Source: three-view drawing plus pictorial views. Frame: mm from the lowest corner of the part. A direction names the side the tool comes from. Give positions to 0.01 mm unless a question says otherwise; leave off trailing zeros. Loops run counter-clockwise (first coordinate to the right, second up) from the corner with the lowest first, then second, coordinate; pieces in that order, holes last. Notation, with made-up numbers: M 78.5,3.25 L 137.5,3.25 A18 cw 137.5,26.25 Z; hole C -30.75,10.5 d6. An arc over 180 degrees is marked long. One line per item, written item: value. Start each with the question number.
(1) Section D-D on z = 28.5. Output: boundary loops of the cut face in (x, y), plus the area to 3 significant figures.
(2) Section B-B on x = 18. Output: boundary loops of the cut face in (y, z).
(3) Section C-C on x = 25. Output: boundary loops of the cut face in (y, z), plus the area to 3 significant figures.
(4) Pin query (flat end, axial travel): P1, Ø6, axis at x = 15, z = 44, coming from the -Y side; P2, Ø1.5, axis at y = 25, z = 49, coming from the -X side; P3, Ø12, axis at y = 7, z = 25.5, coming from the +X side; P4, Ø4.5, axis at y = 5.5, z = 34, coming from the -X side. Return the tip coordinate at first contact, or that it passes through.
(5) Section A-A on z = 16. Output: boundary loops of the cut face in (x, y), plus the area to 3 significant figures.
(6) Ray query, line 1 along X through (y, z) = (42.7, 16); line 2 along Y through (x, z) = (4, 27); line 3 along Z through (x, y) = (18.5, 41.5). Return the intervals inside material, ascending. Write a range as from..to.
(7) Access query for the marked faces 5, 6, 7 and 8. Directions: +Z, -Z, +X, -X, +Y, -Y. A direction counts if a zero-diameter tool reaches every point of the face in a straight line with its end or side. Return the directions, or none.
(8) Pull-direction query (Y, two-part tool) for the marked faces 1, 2, 3 and 4; classes: released by +Y, released by -Y, zero draft, split by the parting line, or undercut.
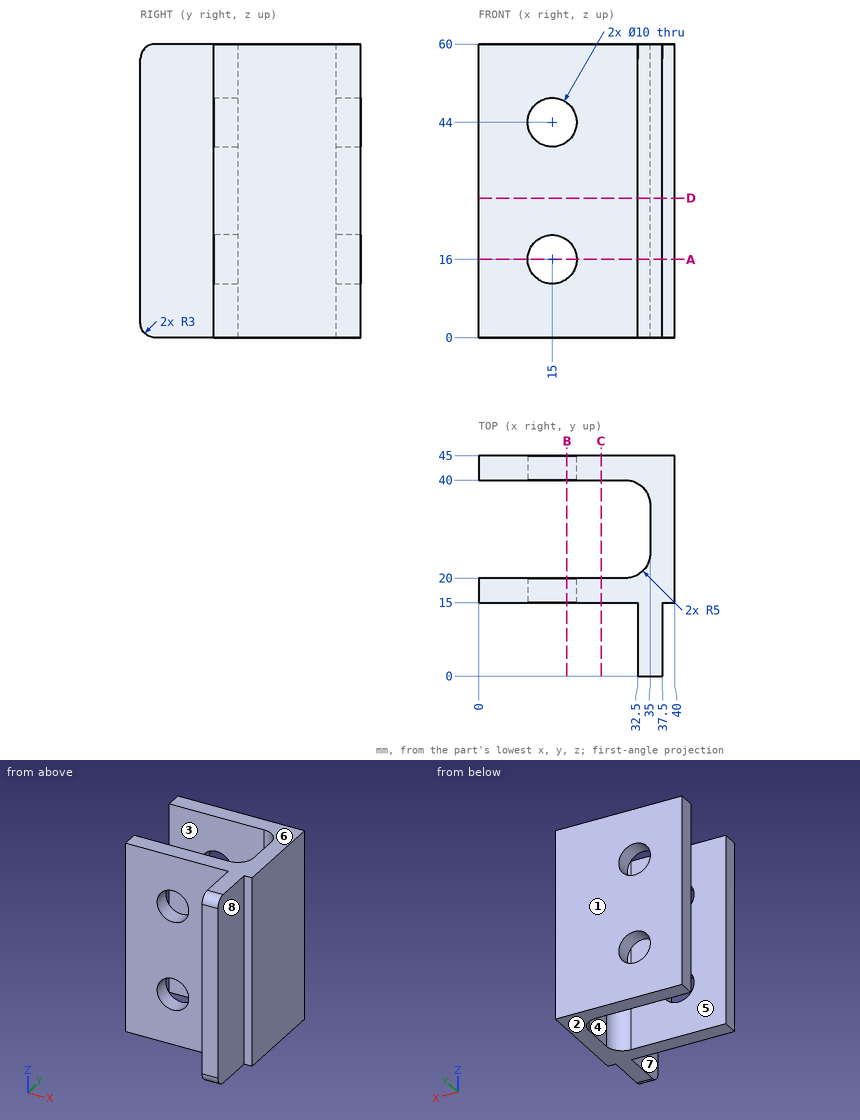
Output values:
1. outline: M 0,15 L 32.5,15 L 32.5,0 L 37.5,0 L 37.5,15 L 40,15 L 40,45 L 0,45 L 0,40 L 30,40 A5 cw 35,35 L 35,25 A5 cw 30,20 L 0,20 Z
1. area: 586 mm²
2. outline: M 15,0 L 20,0 L 20,12 L 15,12 Z; M 15,20 L 20,20 L 20,40 L 15,40 Z; M 15,48 L 20,48 L 20,60 L 15,60 Z; M 40,0 L 45,0 L 45,12 L 40,12 Z; M 40,20 L 45,20 L 45,40 L 40,40 Z; M 40,48 L 45,48 L 45,60 L 40,60 Z
3. outline: M 15,0 L 20,0 L 20,60 L 15,60 Z; M 40,0 L 45,0 L 45,60 L 40,60 Z
3. area: 600 mm²
4. P1: passes through
4. P2: stops at x = 34.94
4. P3: stops at x = 37.5
4. P4: stops at x = 32.5
5. outline: M 0,15 L 10,15 L 10,20 L 0,20 Z; M 0,40 L 10,40 L 10,45 L 0,45 Z; M 20,15 L 32.5,15 L 32.5,0 L 37.5,0 L 37.5,15 L 40,15 L 40,45 L 20,45 L 20,40 L 30,40 A5 cw 35,35 L 35,25 A5 cw 30,20 L 20,20 Z
5. area: 486 mm²
6. line 1: x = 0..10, 20..40
6. line 2: y = 15..20, 40..45
6. line 3: z = 0..12.43, 19.57..40.43, 47.57..60
7. face 5: +Z, -Z, -X
7. face 6: +Z, +X, -X, +Y, -Y
7. face 7: +Z, -Z, -X, -Y
7. face 8: +Z, -Z, +X, -Y
8. face 1: released by +Y
8. face 2: zero draft
8. face 3: undercut
8. face 4: undercut
